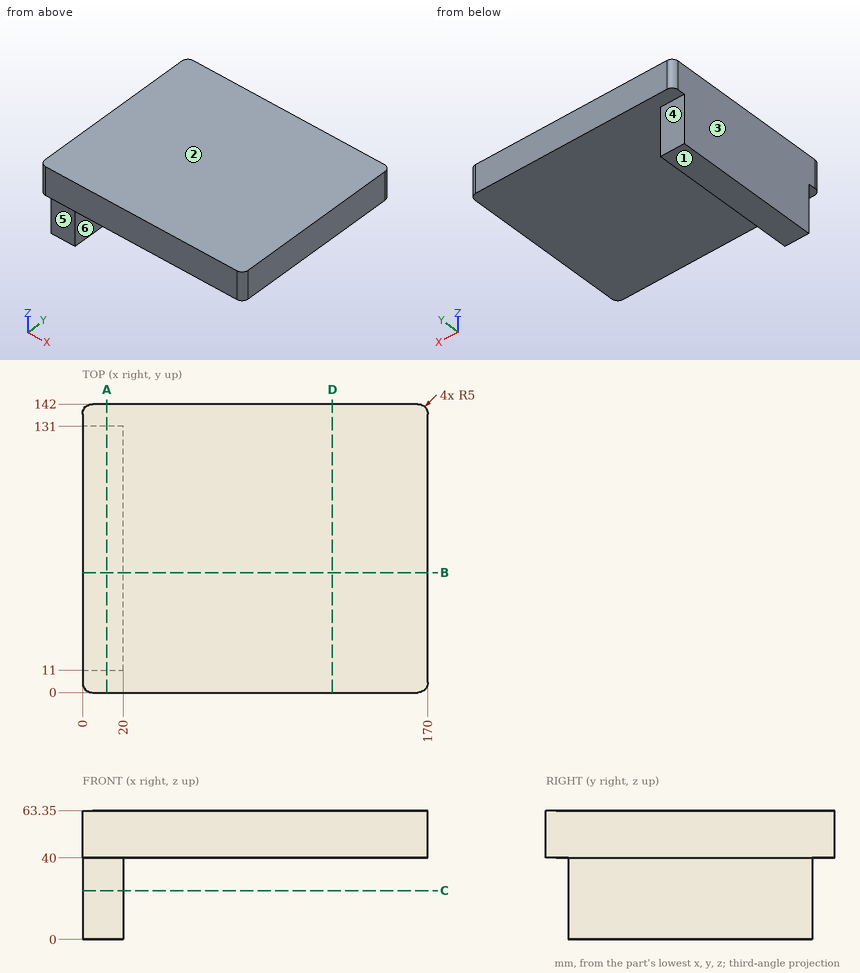
The figure shows three views and two pictorial views of one solid part (mm, origin at its lowest corner). Answer the questions. A direction names the side the tool comes from. Round coordinates to 2 decimals unless told otherwise and drop trailing zeros. Order: outer loops, then holes, each group sorted by start corner. A loop starts at its lowest first (then second) coordinate and runs counter-clockwise, first axis right, second up. Notation, with made-up numbers: M 8.5,80.5 L 30.5,80.5 A22 cw 30.5,102.5 Z; hole C -23.5,55 d6. An arc over 180 degrees is marked long. Answer in a Markdown table with one row per item. Add a question column.
1) The part is cut by section B-B on y = 59. Determine the outline of the cut face in (x, z).
2) The part is cut by section A-A on x = 12. Determine the outline of the cut face in (y, z).
3) Which of the six approach directions +Z, -Z, +X, -X, +Y, -Y give full straight-line access (tool end or side, diameter ignored) to the marked faces 4, 5 and 6?
4) The part is cut by section C-C on z = 24. Determine the outline of the cut face in (x, y).
5) The part is cut by section D-D on x = 123. Determine the outline of the cut face in (y, z).
6) Flat-ended cylindrical pins translate along their axes: pin 1 Ø12 at (y, z) = (44, 12) entering from +X; pin 2 Ø2 at (y, z) = (34.5, 28.5) entering from -X; pin 3 Ø10 at (x, z) = (11.5, 21.5) entering from -Y; pin 4 Ø5 at (x, y) = (104.5, 54) entering from -Z. Find the tip coordinate at first contact, or state that the pin passes through.
7) Consider line 1 along Z through (x, y) = (88, 78.5); line 2 along X through (y, z) = (112.5, 3). Determine where each line is inside the solid, lowest interval first. Write a range as from..to.
8) Determine the mould class of the marked faces 1, 2 and 3 for opening direction Z: pulls with the +Z half, pulls with the -Z half, needs draft (parallel to the pull), parting line crosses it, or undercut.
Findings below:
| question | item | result |
|---|---|---|
| 1 | outline | M 0,0 L 20,0 L 20,40 L 170,40 L 170,63.35 L 0,63.35 Z |
| 2 | outline | M 0,40 L 11,40 L 11,0 L 131,0 L 131,40 L 142,40 L 142,63.35 L 0,63.35 Z |
| 3 | face 4 | -Z, +X, -X, +Y |
| 3 | face 5 | -Z, +X, -X, -Y |
| 3 | face 6 | -Z, +X, +Y, -Y |
| 4 | outline | M 0,11 L 20,11 L 20,131 L 0,131 Z |
| 5 | outline | M 0,40 L 142,40 L 142,63.35 L 0,63.35 Z |
| 6 | pin 1 | stops at x = 20 |
| 6 | pin 2 | stops at x = 0 |
| 6 | pin 3 | stops at y = 11 |
| 6 | pin 4 | stops at z = 40 |
| 7 | line 1 | z = 40..63.35 |
| 7 | line 2 | x = 0..20 |
| 8 | face 1 | pulls with the -Z half |
| 8 | face 2 | pulls with the +Z half |
| 8 | face 3 | needs draft |
